from build123d import *

# Parameters (mm, degrees)
SKETCH_1_W          = 6
SKETCH_1_H          = 30
EXTRUDE_1_DEPTH     = 227
SKETCH_2_R          = 22.5
EXTRUDE_2_DEPTH     = 6
SKETCH_3_R          = 14
CUT_EXTRUDE_1_DEPTH = 231.154839184
HOLE_WIZARD_M32_D   = 3.4
EXTRUDE_3_DEPTH     = 6
HOLE_WIZARD_M31_D   = 3.4
SKETCH_14_W         = 45
SKETCH_14_H         = 6
CUT_EXTRUDE_2_DEPTH = 1
CUT_EXTRUDE_START   = -6
CUT_EXTRUDE_3_DEPTH = 6
CUT_EXTRUDE_5_REACH = 135.036
FILLET_2_R          = 2


with BuildPart() as part:
    # Эскиз1 → Бобышка-Вытянуть1 (new body)
    with BuildSketch(Plane(origin=(0, 0, 0), x_dir=(1, 0, 0), z_dir=(0, 1, 0))):
        with Locations((3, -15)):
            Rectangle(SKETCH_1_W, SKETCH_1_H)
    extrude(amount=EXTRUDE_1_DEPTH)

    # Эскиз2 → Бобышка-Вытянуть2 (add)
    with BuildSketch(Plane.ZY):
        with Locations((15, 105)):
            Circle(SKETCH_2_R)
    extrude(amount=-EXTRUDE_2_DEPTH)

    # Эскиз3 → Вырез-Вытянуть1 (cut, through all)
    with BuildSketch(Plane.ZY):
        with Locations((15, 105)):
            Circle(SKETCH_3_R)
    extrude(amount=-CUT_EXTRUDE_1_DEPTH, mode=Mode.SUBTRACT)

    # Отверстие с зазором M32 (through all)
    with Locations(Plane(origin=(6, -25.024735225, 7.262908886), x_dir=(0, 0, 1), z_dir=(1, 0, 0))):
        with Locations((7.737091114, -149.274735225), (-11.512908886, -130.024735225), (7.737091114, -110.774735225), (26.987091114, -130.024735225)):
            Hole(HOLE_WIZARD_M32_D / 2)

    # Эскиз11 → Бобышка-Вытянуть3 (add)
    with BuildSketch(Plane(origin=(6, 0, 0), x_dir=(0, 0, -1), z_dir=(1, 0, 0))):
        Polygon((0, 18.990381057), (7.5, 6), (7.5, 0), (-37.5, 0), (-37.5, 6), (-30, 18.990381057), align=None)
    extrude(amount=-EXTRUDE_3_DEPTH)

    # Отверстие с зазором M31 (through all)
    with Locations(Plane(origin=(6, 0, 0), x_dir=(0, 0, -1), z_dir=(1, 0, 0))):
        with Locations((-31.875, 3), (-20.625, 3), (-9.375, 3), (1.875, 3)):
            Hole(HOLE_WIZARD_M31_D / 2)

    # Эскиз14 → Вырез-Вытянуть2 (cut)
    with BuildSketch(Plane(origin=(6, 0, 0), x_dir=(0, 0, -1), z_dir=(1, 0, 0))):
        with Locations((-15, 3)):
            Rectangle(SKETCH_14_W, SKETCH_14_H)
    extrude(amount=-CUT_EXTRUDE_2_DEPTH, mode=Mode.SUBTRACT)

    # Эскиз15 → Вырез-Вытянуть3 (cut)
    with BuildSketch(Plane(origin=(6, 0, 0), x_dir=(0, 0, -1), z_dir=(1, 0, 0)).offset(CUT_EXTRUDE_START)):
        with BuildLine():
            Line((-30, 227), (0, 227))
            Line((0, 227), (0, 121.770509831))
            ThreePointArc((0, 121.770509831), (-15, 127.5), (-30, 121.770509831))
            Line((-30, 121.770509831), (-30, 227))
        make_face()
    extrude(amount=CUT_EXTRUDE_3_DEPTH, mode=Mode.SUBTRACT)

    # Эскиз17 → Вырез-Вытянуть5 (cut, up to next)
    with BuildSketch(Plane(origin=(6, 0, 0), x_dir=(0, 0, -1), z_dir=(1, 0, 0)), mode=Mode.PRIVATE) as cut_extrude_5_sk1:
        with BuildLine():
            Line((-17, 82.589065169), (-17, 77.479065169))
            Line((-17, 77.479065169), (-26, 74.203333061))
            Line((-26, 74.203333061), (-26, 85.372213574))
            ThreePointArc((-26, 85.372213574), (-21.647291084, 83.504337153), (-17, 82.589065169))
        make_face()
    cut_extrude_5_tool1 = extrude(cut_extrude_5_sk1.sketch, amount=-CUT_EXTRUDE_5_REACH, mode=Mode.PRIVATE) & part.part
    # Эскиз17 → Вырез-Вытянуть5 (cut, up to next)
    with BuildSketch(Plane(origin=(6, 0, 0), x_dir=(0, 0, -1), z_dir=(1, 0, 0)), mode=Mode.PRIVATE) as cut_extrude_5_sk2:
        with BuildLine():
            Line((-13, 82.589065169), (-13, 77.479065169))
            Line((-13, 77.479065169), (-4, 74.203333061))
            Line((-4, 74.203333061), (-4, 85.372213574))
            ThreePointArc((-4, 85.372213574), (-8.352708916, 83.504337153), (-13, 82.589065169))
        make_face()
    cut_extrude_5_tool2 = extrude(cut_extrude_5_sk2.sketch, amount=-CUT_EXTRUDE_5_REACH, mode=Mode.PRIVATE) & part.part
    # Эскиз17 → Вырез-Вытянуть5 (cut, up to next)
    with BuildSketch(Plane(origin=(6, 0, 0), x_dir=(0, 0, -1), z_dir=(1, 0, 0)), mode=Mode.PRIVATE) as cut_extrude_5_sk3:
        Polygon((-26, 69.946621971), (-15, 73.950294548), (-10.072966814, 72.157001125), (-26, 62.961524227), align=None)
    cut_extrude_5_tool3 = extrude(cut_extrude_5_sk3.sketch, amount=-CUT_EXTRUDE_5_REACH, mode=Mode.PRIVATE) & part.part
    # Эскиз17 → Вырез-Вытянуть5 (cut, up to next)
    with BuildSketch(Plane(origin=(6, 0, 0), x_dir=(0, 0, -1), z_dir=(1, 0, 0)), mode=Mode.PRIVATE) as cut_extrude_5_sk4:
        Polygon((-4, 71.044427996), (-4, 45.641016151), (-26, 58.342722074), align=None)
    cut_extrude_5_tool4 = extrude(cut_extrude_5_sk4.sketch, amount=-CUT_EXTRUDE_5_REACH, mode=Mode.PRIVATE) & part.part
    # Эскиз17 → Вырез-Вытянуть5 (cut, up to next)
    with BuildSketch(Plane(origin=(6, 0, 0), x_dir=(0, 0, -1), z_dir=(1, 0, 0)), mode=Mode.PRIVATE) as cut_extrude_5_sk5:
        Polygon((-26, 53.72391992), (-4, 41.022213998), (-26, 28.320508076), align=None)
    cut_extrude_5_tool5 = extrude(cut_extrude_5_sk5.sketch, amount=-CUT_EXTRUDE_5_REACH, mode=Mode.PRIVATE) & part.part
    # Эскиз17 → Вырез-Вытянуть5 (cut, up to next)
    with BuildSketch(Plane(origin=(6, 0, 0), x_dir=(0, 0, -1), z_dir=(1, 0, 0)), mode=Mode.PRIVATE) as cut_extrude_5_sk6:
        Polygon((-26, 23.701705922), (-4, 36.403411844), (-4, 11), align=None)
    cut_extrude_5_tool6 = extrude(cut_extrude_5_sk6.sketch, amount=-CUT_EXTRUDE_5_REACH, mode=Mode.PRIVATE) & part.part
    # Эскиз17 → Вырез-Вытянуть5 (cut, up to next)
    with BuildSketch(Plane(origin=(6, 0, 0), x_dir=(0, 0, -1), z_dir=(1, 0, 0)), mode=Mode.PRIVATE) as cut_extrude_5_sk7:
        Polygon((-26, 19.082903769), (-12, 11), (-26, 11), align=None)
    cut_extrude_5_tool7 = extrude(cut_extrude_5_sk7.sketch, amount=-CUT_EXTRUDE_5_REACH, mode=Mode.PRIVATE) & part.part
    add(cut_extrude_5_tool1.solids().sort_by_distance((6, 79.721351, 22.080636))[0], mode=Mode.SUBTRACT)
    add(cut_extrude_5_tool2.solids().sort_by_distance((6, 79.721351, 7.919364))[0], mode=Mode.SUBTRACT)
    add(cut_extrude_5_tool3.solids().sort_by_distance((6, 69.313955, 19.731103))[0], mode=Mode.SUBTRACT)
    add(cut_extrude_5_tool4.solids().sort_by_distance((6, 58.342722, 11.333333))[0], mode=Mode.SUBTRACT)
    add(cut_extrude_5_tool5.solids().sort_by_distance((6, 41.022214, 18.666667))[0], mode=Mode.SUBTRACT)
    add(cut_extrude_5_tool6.solids().sort_by_distance((6, 23.701706, 11.333333))[0], mode=Mode.SUBTRACT)
    add(cut_extrude_5_tool7.solids().sort_by_distance((6, 13.694301, 21.333333))[0], mode=Mode.SUBTRACT)

    # Скругление2
    fillet_2_edges = [part.edges().sort_by_distance(p)[0] for p in [
        (3, 88.229490169, 0),
        (3, 85.372213574, 26),
        (3, 82.589065169, 17),
        (3, 77.479065169, 17),
        (3, 74.203333061, 26),
        (3, 82.589065169, 13),
        (3, 85.372213574, 4),
        (3, 74.203333061, 4),
        (3, 77.479065169, 13),
        (3, 62.961524227, 26),
        (3, 69.946621971, 26),
        (3, 73.950294548, 15),
        (3, 72.157001125, 10.072966814),
        (3, 28.320508076, 26),
        (3, 53.72391992, 26),
        (3, 41.022213998, 4),
        (3, 58.342722074, 26),
        (3, 71.044427996, 4),
        (3, 45.641016151, 4),
        (3, 88.229490169, 30),
        (3, 11, 4),
        (3, 23.701705922, 26),
        (3, 36.403411844, 4),
        (3, 11, 26),
        (3, 19.082903769, 26),
        (3, 11, 12),
        (3, 18.990381057, 30),
        (3, 18.990381057, 0),
    ]]
    fillet(fillet_2_edges, radius=FILLET_2_R)


solid = part.part
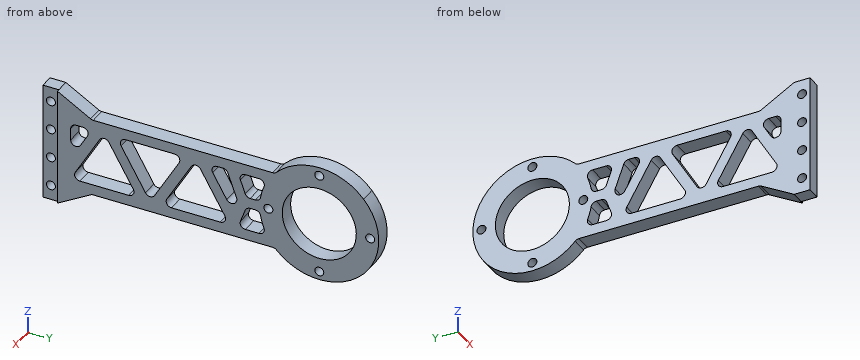
Input: part model. Units: mm. Frame: model coordinates. Coordinates: 2 decimals unless noted, no trailing zeros. Write each loop counter-clockwise with the first axis right and the second up, starting at its lowest first coordinate (ties: lowest second). Pieces come first, ordered by that corner, then holes. Notation, with made-up numbers: M -5.75,-6.5 L 42.25,-6.5 A29 ccw 42.25,24.5 Z; hole C 49.25,43.25 d9. An arc over 180 degrees is marked long. Answer as a JSON object with one key per item and string values. Group by question number.
(1) Ray query, line 1 along Y through (x, z) = (2.5, 32); line 2 along Z through (x, y) = (1.5, 13.5); line 3 along Z through (x, y) = (4, 33.5). Return the intervals inside material, ascending. Write a range as [from, to].
(2) Section C-C on z = 2.5. Output: boundary loops of the cut face in (x, y).
(3) Contact query for flat-ended pins moving along their axis: P1, Ø3, axis at x = 1.5, y = 64.5, coming from the +Z side; P2, Ø3, axis at x = 3.5, y = 41.5, coming from the -Z side; P3, Ø4.5, axis at y = 3, z = -1.875, coming from the +X side; P4, Ø2, axis at y = 3, z = 20.625, coming from the +X side. Output: stop coordinate, or through.
(4) Section B-B on y = 85.75. Output: boundary loops of the cut face in (x, z).
(5) Section A-A on y = 3. Output: boundary loops of the cut face in (x, z) (3 decimals), plus the area to 3 significant figures.
(6) Section D-D on x = 4. Give the number of separate pieces and of enclosed holes in the cut face, plus the area to 3 significant figures.
Result set:
{
 "1": {"line 1": "y = [0, 1.3], [4.7, 15.53], [90.26, 119.74]", "line 2": "z = [-3.17, 4.25], [8.33, 17.53], [26, 33.17]", "line 3": "z = [0, 4.08], [9.03, 17.03], [26, 30]"},
 "2": {"outline": "M 0,0 L 5,0 L 5,6 L 6,6 L 6,98.7 L 0,98.7 Z; M 0,111.3 L 6,111.3 L 6,123.71 L 0,123.71 Z"},
 "3": {"P1": "stops at z = 30", "P2": "stops at z = 0", "P3": "stops at x = 5", "P4": "passes through"},
 "4": {"outline": "M 0,0 L 6,0 L 6,13.3 L 0,13.3 Z; M 0,16.7 L 6,16.7 L 6,30 L 0,30 Z"},
 "5": {"outline": "M 0,-7.5 L 5,-7.5 L 5,-3.575 L 0,-3.575 Z; M 0,-0.175 L 5,-0.175 L 5,7.675 L 0,7.675 Z; M 0,11.075 L 5,11.075 L 5,18.925 L 0,18.925 Z; M 0,22.325 L 5,22.325 L 5,30.175 L 0,30.175 Z; M 0,33.575 L 5,33.575 L 5,37.5 L 0,37.5 Z", "area": "157 mm2"},
 "6": {"separate pieces": "1", "enclosed holes": "16", "area": "2,560 mm2"}
}
